from build123d import *

# Parameters (mm, degrees)
SKETCH2_R           = 5.0419
SKETCH2_R_2         = 3.3782
BOSS_EXTRUDE2_DEPTH = 3.175
SKETCH3_R           = 3.3782
SKETCH3_R_2         = 2.54
CUT_EXTRUDE1_DEPTH  = 408.087553815
CHAMFER1_SIZE       = 3.175
FILLET1_R           = 25.4


with BuildPart() as part:
    # Sketch2 → Boss-Extrude2 (new body)
    with BuildSketch(Plane(origin=(0, 0, 0), x_dir=(0, 0, -1), z_dir=(1, 0, 0))):
        with BuildLine():
            Line((25.4, 0), (25.4, 25.4))
            Line((25.4, 25.4), (49.872202827, 370.551588468))
            ThreePointArc((49.872202827, 370.551588468), (61.818783569, 382.33286047), (75.02488963, 371.98308153))
            Line((75.02488963, 371.98308153), (139.7, 25.4))
            Line((139.7, 25.4), (139.7, 0))
            Line((139.7, 0), (25.4, 0))
        make_face()
        with Locations((63.5, 82.55)):
            Circle(SKETCH2_R, mode=Mode.SUBTRACT)
        with Locations((62.540399951, 369.653378233)):
            Circle(SKETCH2_R_2, mode=Mode.SUBTRACT)
    extrude(amount=BOSS_EXTRUDE2_DEPTH)

    # Sketch3 → Cut-Extrude1 (cut, through all)
    with BuildSketch(Plane(origin=(3.175, 0, 0), x_dir=(0, 0, -1), z_dir=(1, 0, 0))):
        with Locations((38.1, 12.7)):
            Circle(SKETCH3_R)
        with Locations((82.55, 12.7)):
            Circle(SKETCH3_R)
        with Locations((127, 12.7)):
            Circle(SKETCH3_R)
        with Locations((93.193559072, 240.004229778)):
            Circle(SKETCH3_R_2)
        with Locations((115.586891115, 120.002114889)):
            Circle(SKETCH3_R_2)
    extrude(amount=-CUT_EXTRUDE1_DEPTH, mode=Mode.SUBTRACT)

    # Chamfer1
    chamfer1_edges = [part.edges().sort_by_distance(p)[0] for p in [
        (1.5875, 0, -25.4),
        (1.5875, 0, -139.7),
    ]]
    chamfer(chamfer1_edges, length=CHAMFER1_SIZE)

    # Fillet1
    # the kernel refuses this fillet: 25.4 mm, written as the material it takes off along each edge
    with BuildSketch(Plane(origin=(-2.248340694, 25.4, -25.4), x_dir=(0, -1, 0), z_dir=(1, 0, 0))) as fillet1_piece_1:
        with BuildLine():
            CenterArc((FILLET1_R * 0.0354069400697, FILLET1_R), FILLET1_R, 265.944357758, 4.055642242)
            Line((-FILLET1_R * 0.0353182753041, FILLET1_R * 0.00250416346216), (0, 0))
            Line((0, 0), (FILLET1_R * 0.0354069400697, 0))
        make_face()
    extrude(amount=7.671681389, mode=Mode.SUBTRACT)
    with BuildSketch(Plane(origin=(-5.874097958, 25.4, -139.7), x_dir=(0, 0.9830306833875174, 0.1834412045279636), z_dir=(1, 0, 0))) as fillet1_piece_2:
        with BuildLine():
            CenterArc((FILLET1_R * 0.0925054796503, FILLET1_R), FILLET1_R, 259.429735221, 10.570264779)
            Line((-FILLET1_R * 0.0909357248777, FILLET1_R * 0.0169693166125), (0, 0))
            Line((0, 0), (FILLET1_R * 0.0925054796503, 0))
        make_face()
    extrude(amount=14.923195916, mode=Mode.SUBTRACT)


solid = part.part
Input: part model. Units: mm. Frame: model coordinates. Coordinates: 2 decimals unless noted, no trailing zeros. Order: outer loops, then holes, each group sorted by start corner. A loop starts at its lowest first (then second) coordinate and runs counter-clockwise, first axis right, second up.
1. Contact query for a flat-ended pin moving along its axis: P1, Ø3, axis at y = 240, z = -93.19, coming from the +X side. Output: stop coordinate, or through.
Checked values:
P1: passes through
2. Cut plane D-D, the plane y = 82.55. Return loops of the section in (x, z) (3 decimals), plus the area to 3 significant figures.
Checked values:
outline: (0, -129.035) - (3.175, -129.035) - (3.175, -68.542) - (0, -68.542) - close; (0, -58.458) - (3.175, -58.458) - (3.175, -29.452) - (0, -29.452) - close
area: 284 mm2
3. Cut plane C-C, the plane z = -127. Return loops of the section in (x, y) (3 decimals), plus the area to 3 significant figures.
Checked values:
outline: (0, 0) - (3.175, 0) - (3.175, 9.322) - (0, 9.322) - close; (0, 16.078) - (3.175, 16.078) - (3.175, 93.457) - (0, 93.457) - close
area: 275 mm2
4. Ray query, line 1 along Y through (x, z) = (1.55, -63.5); line 2 along Y through (x, z) = (1.35, -62); line 3 along Z through (x, y) = (1.6, 209). Return the intervals inside material, ascending.
Checked values:
line 1: y = 0 to 77.51, 87.59 to 366.41, 372.89 to 382.32
line 2: y = 0 to 77.74, 87.36 to 366.32, 372.99 to 382.34
line 3: z = -105.44 to -38.42
5. Draft query along Z for faces 1 (the cylindrical face through (1.61, 11.406, -85.671)), 2 (the flat face through (3.175, 151, -71)), 3 (the cylindrical face through (1.565, 382.316, -61.563)). Return one class per face: +Z half, -Z half, draft (parallel to the pull), parting line (faces both ways), or undercut.
Checked values:
face 1: undercut
face 2: draft
face 3: parting line
6. Cut plane A-A, the plane y = 12.7. Return loops of the section in (x, z) (3 decimals), plus the area to 3 significant figures.
Checked values:
outline: (0, -139.7) - (3.175, -139.7) - (3.175, -130.378) - (0, -130.378) - close; (0, -123.622) - (3.175, -123.622) - (3.175, -85.928) - (0, -85.928) - close; (0, -79.172) - (3.175, -79.172) - (3.175, -41.478) - (0, -41.478) - close; (0, -34.722) - (3.175, -34.722) - (3.175, -25.4) - (0, -25.4) - close
area: 299 mm2
7. Cut plane B-B, the plane x = 0.85. Return loops of the section in (y, z) (3 decimals), plus the area to 3 significant figures.
Checked values:
outline: (0, -136.525) - (3.175, -139.7) - (23.05, -139.7) arc R25.4 ccw to (27.71, -139.269) - (371.983, -75.025) arc R12.7 ccw to (370.552, -49.872) - (26.297, -25.464) arc R25.4 ccw to (24.501, -25.4) - (3.175, -25.4) - (0, -28.575) - close; hole circle Ø6.756 at (12.7, -127); hole circle Ø6.756 at (12.7, -82.55); hole circle Ø6.756 at (12.7, -38.1); hole circle Ø10.084 at (82.55, -63.5); hole circle Ø5.08 at (120.002, -115.587); hole circle Ø5.08 at (240.004, -93.194); hole circle Ø6.756 at (369.653, -62.54)
area: 27,000 mm2
